Work out the finished part from the listing and answer in its coordinate system (mm). A direction names the side the tool comes from. Coordinates: 2 decimals unless noted, no trailing zeros. Loops run counter-clockwise (first coordinate to the right, second up) from the corner with the lowest first, then second, coordinate; pieces in that order, holes last.
```python
from build123d import *

# Parameters (mm, degrees)
CHAMFER2_SIZE      = 2.38
CUT_EXTRUDE1_START = -12.7
SKETCH2_R          = 6.35
SKETCH2_R_2        = 3.902029093
CUT_EXTRUDE1_DEPTH = 12.7


with BuildPart() as part:
    # Sketch1 → Revolve1 (revolve)
    with BuildSketch(Plane.XY, mode=Mode.PRIVATE) as revolve1_sk:
        with BuildLine():
            Line((0, 248.389026298), (6.35, 248.389026298))
            Line((6.35, 248.389026298), (6.35, 222.989026298))
            ThreePointArc((6.35, 222.989026298), (28.800640303, 213.6896666), (38.1, 191.239026298))
            Line((38.1, 191.239026298), (38.1, -18.310973702))
            Line((38.1, -18.310973702), (0, -18.310973702))
            Line((0, -18.310973702), (0, 248.389026298))
        make_face()
    revolve(revolve1_sk.sketch.rotate(Axis((0, 337.108439078, 0), (0, -1, 0)), 90), axis=Axis((0, 337.108439078, 0), (0, -1, 0)))

    # Chamfer2
    # the kernel refuses this chamfer: 2.38 mm, written as the material it adds along each edge
    with BuildSketch(Plane(origin=(0, 222.989026298, 0), x_dir=(0, 0, 1), z_dir=(1, 0, 0))) as chamfer2_piece_1:
        with BuildLine():
            Line((6.35, -CHAMFER2_SIZE), (8.826750448, 0.096750448))
            ThreePointArc((8.826750448, 0.096750448), (7.624301016, 0.025582639), (6.35, 0))
            Line((6.35, 0), (6.35, -CHAMFER2_SIZE))
        make_face()
    revolve(axis=Axis((0, 222.989026298, 0), (0, -1, 0)))

    # Sketch2 → Cut-Extrude1 (cut)
    with BuildSketch(Plane(origin=(0, 248.389026298, 0), x_dir=(1, 0, 0), z_dir=(0, 1, 0)).offset(CUT_EXTRUDE1_START)):
        with Locations(Location((0, 0, 0), (0, 0, 270))):
            Circle(SKETCH2_R)
        with Locations(Location((0, 0, 0), (0, 0, 270))):
            Circle(SKETCH2_R_2, mode=Mode.SUBTRACT)
    extrude(amount=CUT_EXTRUDE1_DEPTH, mode=Mode.SUBTRACT)


solid = part.part
```
1. A cutting plane is placed at B-B, the plane y = 95. Give the vertices of the cut face in (x, z).
2. Straight lines are drawn through the part: probe 1 along Z at (x, y) = (2, 123); probe 2 along Z at (x, y) = (19, 180.5); probe 3 along Y at (x, z) = (28.5, 5). For each, find the intervals that lie inside material, in ascending order.
3. Each of these flat-tipped pins is pushed along its axis until it touches: P1, Ø10, axis at y = 165.5, z = 8, coming from the +X side; P2, Ø2, axis at x = 13, y = 44.5, coming from the -Z side; P3, Ø1, axis at x = 13.5, z = -21, coming from the +Y side; P4, Ø10, axis at x = -3.5, y = 44, coming from the -Z side. Where does it stop, or does it pass through?
4. For faces 1 (the cylindrical face through (-1.495, 241.95, 3.604)), 2 (the flat face through (0, 248.389, 0)), determine the directions among +Z, -Z, +X, -X, +Y, -Y from which every point of the face is accessible in a straight line to the end or side of a thin tool.
5. A cutting plane is placed at A-A, the plane y = 232. Give the vertices of the cut face in (x, z).
Answers below:
1. outline: circle Ø76.2 at (0, 0)
2. probe 1: z = -38.05 to 38.05
2. probe 2: z = -33.02 to 33.02
2. probe 3: y = -18.31 to 213.55
3. P1: stops at x = 37.98
3. P2: stops at z = -36.16
3. P3: stops at y = 217.31
3. P4: stops at z = -38.1
4. face 1: +Y
4. face 2: +Z, -Z, +X, -X, +Y
5. outline: circle Ø12.7 at (0, 0)
